CAD build for the part. Positions are in the model's coordinates, mm. Face numbers are marked on the shaded views. A direction names the side the tool comes from. Round coordinates to 2 decimals unless told otherwise and drop trailing zeros. Order: outer loops, then holes, each group sorted by start corner. A loop starts at its lowest first (then second) coordinate and runs counter-clockwise, first axis right, second up. Notation, with made-up numbers: M 40,64 L 55,64 A16 ccw 55,72 Z; hole C 68,41 d10. An arc over 180 degrees is marked long. Put each result on its own line as item: value.
```python
from build123d import *

# Parameters (mm, degrees)
SKETCH1_W           = 20
SKETCH1_H           = 54
BOSS_EXTRUDE1_DEPTH = 2
SKETCH2_W           = 20
SKETCH2_H           = 2
BOSS_EXTRUDE2_DEPTH = 50
FILLET1_R           = 1
SKETCH3_W           = 2
SKETCH3_H           = 43.466929313
BOSS_EXTRUDE3_DEPTH = 40
SKETCH4_R           = 2.5
CUT_EXTRUDE1_DEPTH  = 78.588658965


with BuildPart() as part:
    # Sketch1 → Boss-Extrude1 (new body)
    with BuildSketch(Plane.XY):
        with Locations((10, 27)):
            Rectangle(SKETCH1_W, SKETCH1_H)
    extrude(amount=BOSS_EXTRUDE1_DEPTH)

    # Sketch2 → Boss-Extrude2 (add)
    with BuildSketch(Plane.XY.offset(2)):
        with Locations((10, 53)):
            Rectangle(SKETCH2_W, SKETCH2_H)
        with Locations((10, 1)):
            Rectangle(SKETCH2_W, SKETCH2_H)
    extrude(amount=BOSS_EXTRUDE2_DEPTH)

    # Fillet1
    fillet1_edges = [part.edges().sort_by_distance(p)[0] for p in [
        (10, 54, 0),
        (10, 0, 0),
    ]]
    fillet(fillet1_edges, radius=FILLET1_R)

    # Sketch3 → Boss-Extrude3 (add)
    with BuildSketch(Plane(origin=(0, 0, 0), x_dir=(-1, 0, 0), z_dir=(0, 0, -1))):
        with Locations((-19, 26.891060328)):
            Rectangle(SKETCH3_W, SKETCH3_H)
        with Locations((-1, 26.891060328)):
            Rectangle(SKETCH3_W, SKETCH3_H)
    extrude(amount=BOSS_EXTRUDE3_DEPTH)

    # Sketch4 → Cut-Extrude1 (cut, through all)
    with BuildSketch(Plane(origin=(20, 0, 0), x_dir=(0, 0, -1), z_dir=(1, 0, 0))):
        with Locations((23.160609429, 26.891060328)):
            Circle(SKETCH4_R)
    extrude(amount=-CUT_EXTRUDE1_DEPTH, mode=Mode.SUBTRACT)


solid = part.part
```
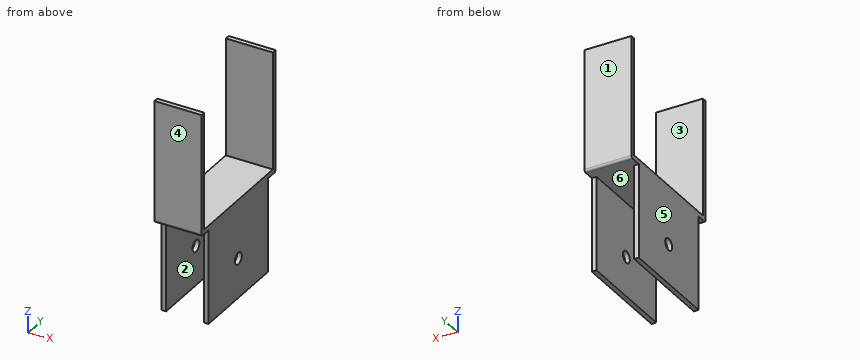
Item 1: Band-saw the part on D-D on z = 36. Give the cut face in (x, y), and give its area (3 significant figures).
Answers below:
outline: M 0,0 L 20,0 L 20,2 L 0,2 Z; M 0,52 L 20,52 L 20,54 L 0,54 Z
area: 80.0 mm²
Item 2: Tool access for the marked faces 1, 2 and 3: list every direction of +Z, -Z, +X, -X, +Y, -Y with a clear straight run to the whole face (end or side of a thin tool).
Answers below:
face 1: +Z, -Z, +X, -X, +Y
face 2: -Z, +Y, -Y
face 3: +Z, +X, -X
Item 3: Probe line 1 along X through (y, z) = (33.5, -1); line 2 along Y through (x, z) = (17, 27); line 3 along Z through (x, y) = (16, 39). List the from-to ranges inside material, lowest first. Write a range as [from, to].
Answers below:
line 1: [0, 2], [18, 20]
line 2: [0, 2], [52, 54]
line 3: [0, 2]
Item 4: Band-saw the part on B-B on x = 10. Give the cut face in (y, z).
Answers below:
outline: M 0,1 A1 ccw 1,0 L 53,0 A1 ccw 54,1 L 54,52 L 52,52 L 52,2 L 2,2 L 2,52 L 0,52 Z
Item 5: Band-saw the part on C-C on y = 46. Give the cut face in (x, z), and give its area (3 significant figures).
Answers below:
outline: M 0,-40 L 2,-40 L 2,0 L 18,0 L 18,-40 L 20,-40 L 20,2 L 0,2 Z
area: 200 mm²
Item 6: Band-saw the part on A-A on z = -10.5. Give the cut face in (x, y), and give its area (3 significant figures).
Answers below:
outline: M 0,5.16 L 2,5.16 L 2,48.62 L 0,48.62 Z; M 18,5.16 L 20,5.16 L 20,48.62 L 18,48.62 Z
area: 174 mm²
Item 7: Pin check, flat tips, straight feed: P1, Ø1.5, axis at x = 7.5, y = 36, coming from the -Z side; P2, Ø4, axis at x = 13, y = 7.5, coming from the +Z side; P3, Ø10, axis at x = 6, y = 10.5, coming from the -Z side; P4, Ø1.6, axis at x = 0.5, z = -14, coming from the +Y side. Stop position of each tip, or through.
Answers below:
P1: z = 0
P2: z = 2
P3: z = -40
P4: y = 48.62
Item 8: Mould opens along X. For the marked faces 4, 5 and 6 say: pulls with the +X half, pulls with the -X half, needs draft (parallel to the pull), parting line crosses it, or undercut.
Answers below:
face 4: needs draft
face 5: pulls with the -X half
face 6: undercut
